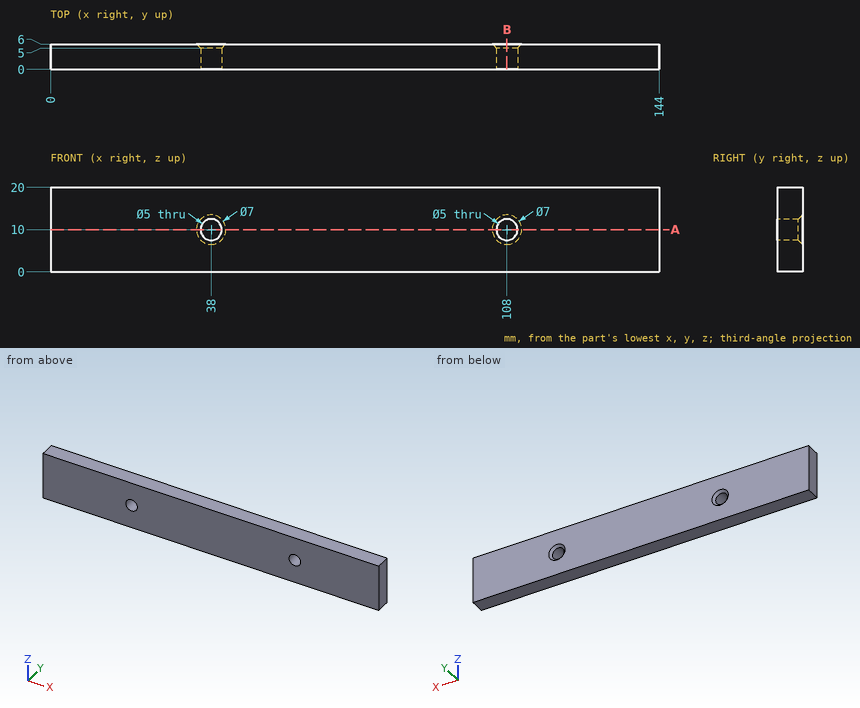
Verification items for this drawing (mm, ordinates from the low corner). Round coordinates to 2 decimals unless told otherwise and drop trailing zeros. Loops run counter-clockwise (first coordinate to the right, second up) from the corner with the lowest first, then second, coordinate; pieces in that order, holes last. Notation, with made-up numbers: (88.5, 18) -> (123.5, 18) arc R26 ccw to (123.5, 54) -> close; hole circle Ø10 at (54.5, -0.5). An arc over 180 degrees is marked (long way). Write item = value, one per line. Start each with the question number.
1) Sectioned sample at A-A, the plane z = 10. Record the cut outline in (x, y).
2) Sectioned sample at B-B, the plane x = 108. Record the cut outline in (y, z).
3) Thickness scan on probe 1 along X at (y, z) = (4.45, 10); probe 2 along Z at (x, y) = (108, 1.5); probe 3 along X at (y, z) = (5.65, 10.25). Record the ranges inside material, lowest first.
Results are:
q1.outline = (0, 0) -> (35.5, 0) -> (35.5, 5) -> (34.5, 6) -> (0, 6) -> close; (40.5, 0) -> (105.5, 0) -> (105.5, 5) -> (104.5, 6) -> (41.5, 6) -> (40.5, 5) -> close; (110.5, 0) -> (144, 0) -> (144, 6) -> (111.5, 6) -> (110.5, 5) -> close
q2.outline = (0, 0) -> (6, 0) -> (6, 6.5) -> (5, 7.5) -> (0, 7.5) -> close; (0, 12.5) -> (5, 12.5) -> (6, 13.5) -> (6, 20) -> (0, 20) -> close
q3.probe_1 = 0 to 35.5, 40.5 to 105.5, 110.5 to 144
q3.probe_2 = 0 to 7.5, 12.5 to 20
q3.probe_3 = 0 to 34.86, 41.14 to 104.86, 111.14 to 144
